```python
from build123d import *

# Parameters (mm, degrees)
SKETCH_1_R      = 20
EXTRUDE_1_DEPTH = 145
SKETCH_2_R      = 17.5
EXTRUDE_2_DEPTH = 8
CHAMFER_2_SIZE  = 3
CHAMFER_1_SIZE  = 1


with BuildPart() as part:
    # 草图1 → 凸台-拉伸1 (new body)
    with BuildSketch(Plane(origin=(0, 0, 0), x_dir=(0, 0, -1), z_dir=(1, 0, 0))):
        Circle(SKETCH_1_R)
    extrude(amount=EXTRUDE_1_DEPTH)

    # 草图2 → 凸台-拉伸2 (add)
    with BuildSketch(Plane.ZY):
        Circle(SKETCH_2_R)
    extrude(amount=EXTRUDE_2_DEPTH)

    # 倒角2
    chamfer_2_edges = [part.edges().sort_by_distance(p)[0] for p in [
        (-8, 0, -17.5),
    ]]
    chamfer(chamfer_2_edges, length=CHAMFER_2_SIZE)

    # 倒角1
    chamfer_1_edges = [part.edges().sort_by_distance(p)[0] for p in [
        (145, 0, 20),
    ]]
    chamfer(chamfer_1_edges, length=CHAMFER_1_SIZE)


solid = part.part
```
CAD build for the part. Positions are in the model's coordinates, mm. A direction names the side the tool comes from. Coordinates: 2 decimals unless noted, no trailing zeros. Order: outer loops, then holes, each group sorted by start corner. A loop starts at its lowest first (then second) coordinate and runs counter-clockwise, first axis right, second up. Notation, with made-up numbers: M 53,77.25 L 98,77.25 A28 ccw 98,116.25 Z; hole C 71,-13 d10. An arc over 180 degrees is marked long. Write each question's results on one line, items separated by ' | '. Start each with the question number.
Q1. Drill centre lines: probe 1 along X at (y, z) = (0, -18); probe 2 along Y at (x, z) = (118.5, 1). Where is each one in solid material? Low to high. Write a range as from..to.
Q2. Which spindle directions (+Z, -Z, +X, -X, +Y, -Y) get a long thin tool onto all of the face, cutting with end or side? Do faces 1 (the flat face through (0, -18, 0)), 2 (the flat face through (-8, 0, 0)). Say none if no direction does.
Q3. Flat gauge pins, fed straight in: P1, Ø4, axis at x = 64, z = -5.5, coming from the -Y side; P2, Ø1.5, axis at x = 79, y = 10.5, coming from the -Z side; P3, Ø1.5, axis at x = 106, y = 12.5, coming from the -Z side; P4, Ø1, axis at x = 129.5, y = 0.5, coming from the +Z side. Where does each tip first touch, or does it go through?
Q4. Cut at A-A (x = 61.5). List the corners of the cut face in (y, z), then the cut area to 3 significant figures.
Found:
1) probe 1: 0..145 | probe 2: -19.97..19.97
2) face 1: -X | face 2: +Z, -Z, -X, +Y, -Y
3) P1: y = -19.69 | P2: z = -17.46 | P3: z = -16.18 | P4: z = 20
4) outline: C 0,0 d40 | area: 1,260 mm²
